For this review, take the finished solid that the model builds, in its own axes (mm). A direction names the side the tool comes from. Coordinates: 2 decimals unless noted, no trailing zeros. Write each loop counter-clockwise with the first axis right and the second up, starting at its lowest first coordinate (ties: lowest second). Pieces come first, ordered by that corner, then holes.
1) We need section B-B on x = 0. Write out the cut boundary in (y, z).
2) We need section C-C on z = -7. Write out the cut boundary in (x, y).
3) For faces 1 (the face through (7.15, -13.59, 48.03)), 2 (the face through (-23, -23, 0)), 3 (the face through (44, 0, -13)), list the 3-axis set-ups (+Z, -Z, +X, -X, +Y, -Y) from which the entire face can be reached by the end or side of a thin tool; tool diameter is ignored.
4) We need section A-A on y = 0. Write out the cut boundary in (x, z), then the cut area to 3 significant figures.
5) To check wall thickness, follow line 1 along Z through (x, y) = (1, -38); line 2 along X through (y, z) = (-0.5, -3); line 3 along Y through (x, z) = (-17.25, 47.6). State the ranges of each line that lie inside material, in increasing order.
6) Insertion check: P1, Ø3.5, axis at x = -8.62, y = -14.94, coming from the -Z side; P2, Ø4.5, axis at x = -42, y = 0, coming from the +Z side; P3, Ø4.5, axis at x = -17.25, y = 0, coming from the -Z side; P4, Ø5, axis at y = -6.5, z = 21, coming from the -X side. Each pin has a flat end and moves straight along its axis. Give the tip position at first contact, or say it passes through.
7) We need section D-D on x = -17.25. Write out the cut boundary in (y, z), then the cut area to 3 significant figures.
from build123d import *

# Parameters (mm, degrees)
SKETCH_1_R          = 29.5
EXTRUDE_1_DEPTH     = 50
SHELL_2_T           = -4
SKETCH_3_R          = 2
CUT_EXTRUDE_1_DEPTH = 66.119121616
SKETCH_5_R          = 54.5
SKETCH_5_R_2        = 29.5
SKETCH_5_R_3        = 25.5
EXTRUDE_7_DEPTH     = 15
SKETCH_6_R          = 2
CUT_EXTRUDE_3_DEPTH = 4


with BuildPart() as part:
    # 草图1 → 凸台-拉伸1 (new body)
    with BuildSketch(Plane.XY):
        Circle(SKETCH_1_R)
    extrude(amount=EXTRUDE_1_DEPTH)

    # 抽壳2
    shell_2_openings = [part.faces().sort_by_distance(p)[0] for p in [
        (0, 0, 0),
    ]]
    offset(amount=SHELL_2_T, openings=shell_2_openings, kind=Kind.INTERSECTION)

    # 草图3 → 切除-拉伸1 (cut, through all)
    with BuildSketch(Plane.XY.offset(50)):
        with Locations((-17.25, 0)):
            Circle(SKETCH_3_R)
        with Locations((-8.625, 14.938938215)):
            Circle(SKETCH_3_R)
        with Locations((8.625, 14.938938215)):
            Circle(SKETCH_3_R)
        with Locations((17.25, 0)):
            Circle(SKETCH_3_R)
        with Locations((8.625, -14.938938215)):
            Circle(SKETCH_3_R)
        with Locations((-8.625, -14.938938215)):
            Circle(SKETCH_3_R)
    extrude(amount=-CUT_EXTRUDE_1_DEPTH, mode=Mode.SUBTRACT)

    # 草图5 → 凸台-拉伸7 (add)
    with BuildSketch(Plane(origin=(0, 0, 0), x_dir=(-1, 0, 0), z_dir=(0, 0, -1))):
        Circle(SKETCH_5_R)
        with Locations(Location((0, 0, 0), (0, 0, 180))):
            Circle(SKETCH_5_R_2, mode=Mode.SUBTRACT)
        with Locations(Location((0, 0, 0), (0, 0, 180))):
            Circle(SKETCH_5_R_2)
        Circle(SKETCH_5_R_3, mode=Mode.SUBTRACT)
    extrude(amount=EXTRUDE_7_DEPTH)

    # 草图6 → 切除-拉伸3 (cut)
    with BuildSketch(Plane(origin=(0, 0, -15), x_dir=(-1, 0, 0), z_dir=(0, 0, -1))):
        with Locations((-42, 0)):
            Circle(SKETCH_6_R)
        with Locations((42, 0)):
            Circle(SKETCH_6_R)
    extrude(amount=-CUT_EXTRUDE_3_DEPTH, mode=Mode.SUBTRACT)


solid = part.part
Result:
1. outline: (-54.5, -15) - (-25.5, -15) - (-25.5, 46) - (25.5, 46) - (25.5, -15) - (54.5, -15) - (54.5, 0) - (29.5, 0) - (29.5, 50) - (-29.5, 50) - (-29.5, 0) - (-54.5, 0) - close
2. outline: circle Ø109 at (0, 0); hole circle Ø51 at (0, 0)
3. face 1: +Z, -Z
3. face 2: +Z
3. face 3: -Z
4. outline: (-54.5, -15) - (-44, -15) - (-44, -11) - (-40, -11) - (-40, -15) - (-25.5, -15) - (-25.5, 46) - (-19.25, 46) - (-19.25, 50) - (-29.5, 50) - (-29.5, 0) - (-54.5, 0) - close; (-15.25, 46) - (15.25, 46) - (15.25, 50) - (-15.25, 50) - close; (19.25, 46) - (25.5, 46) - (25.5, -15) - (40, -15) - (40, -11) - (44, -11) - (44, -15) - (54.5, -15) - (54.5, 0) - (29.5, 0) - (29.5, 50) - (19.25, 50) - close
4. area: 1,410 mm2
5. line 1: z = -15 to 0
5. line 2: x = -54.5 to -25.5, 25.5 to 54.5
5. line 3: y = -23.93 to -2, 2 to 23.93
6. P1: passes through
6. P2: stops at z = 0
6. P3: stops at z = 46
6. P4: stops at x = -29.23
7. outline: (-51.7, -15) - (-18.78, -15) - (-18.78, 46) - (-2, 46) - (-2, 50) - (-23.93, 50) - (-23.93, 0) - (-51.7, 0) - close; (2, 46) - (18.78, 46) - (18.78, -15) - (51.7, -15) - (51.7, 0) - (23.93, 0) - (23.93, 50) - (2, 50) - close
7. area: 1,640 mm2
